Can you work these out from the model? Positions are in its coordinate system, mm. Round coordinates to 2 decimals unless told otherwise and drop trailing zeros.
(1) If I drill on line 1 along Y through (x, z) = (11.6, -881.5) (3 decimals); line 2 along X through (y, z) = (-26.5, -954); line 3 along X through (y, z) = (-21.5, -768), over which ranges is the centre line in solid material (lowest first)?
(2) I want a section at A-A on z = -800. Give the number of separate pieces and of enclosed holes in the cut face, plus the area to 3 significant figures.
(3) Will these pins go through, and if not, where does the flat tip stop? pin 1 Ø0.5 at (x, z) = (13.5, -813) entering from +Y; pin 2 Ø5.5 at (x, y) = (-11.6, -26.625) entering from +Z; pin 3 Ø0.8 at (x, z) = (14, -592) entering from -Y.
from build123d import *

# Parameters (mm, degrees)
SKETCH1_R           = 2.1
SKETCH1_R_2         = 3.4
BOSS_EXTRUDE1_DEPTH = 550


with BuildPart() as part:
    # Sketch1 → Boss-Extrude1 (new body)
    with BuildSketch(Plane(origin=(0, 0, -1000), x_dir=(-1, 0, 0), z_dir=(0, 0, -1))):
        with BuildLine():
            Line((15, -28), (15, -19.3))
            ThreePointArc((15, -19.3), (14.912132034, -19.087867966), (14.7, -19))
            Line((14.7, -19), (13, -19))
            Line((13, -19), (13, -23.25))
            Line((13, -23.25), (9.6642, -23.25))
            Line((9.6642, -23.25), (6, -19.5858))
            Line((6, -19.5858), (6, -15.519615242))
            Line((6, -15.519615242), (5.7, -15))
            Line((5.7, -15), (6, -14.480384758))
            Line((6, -14.480384758), (6, -10.4142))
            Line((6, -10.4142), (9.6642, -6.75))
            Line((9.6642, -6.75), (13, -6.75))
            Line((13, -6.75), (13, -11))
            Line((13, -11), (14.7, -11))
            ThreePointArc((14.7, -11), (14.912132034, -10.912132034), (15, -10.7))
            Line((15, -10.7), (15, 10.7))
            ThreePointArc((15, 10.7), (14.912132034, 10.912132034), (14.7, 11))
            Line((14.7, 11), (13, 11))
            Line((13, 11), (13, 6.75))
            Line((13, 6.75), (9.6642, 6.75))
            Line((9.6642, 6.75), (6, 10.4142))
            Line((6, 10.4142), (6, 14.480384758))
            Line((6, 14.480384758), (5.7, 15))
            Line((5.7, 15), (6, 15.519615242))
            Line((6, 15.519615242), (6, 19.5858))
            Line((6, 19.5858), (9.6642, 23.25))
            Line((9.6642, 23.25), (13, 23.25))
            Line((13, 23.25), (13, 19))
            Line((13, 19), (14.7, 19))
            ThreePointArc((14.7, 19), (14.912132034, 19.087867966), (15, 19.3))
            Line((15, 19.3), (15, 28))
            ThreePointArc((15, 28), (14.414213562, 29.414213562), (13, 30))
            Line((13, 30), (4.3, 30))
            ThreePointArc((4.3, 30), (4.087867966, 29.912132034), (4, 29.7))
            Line((4, 29.7), (4, 28))
            Line((4, 28), (8.25, 28))
            Line((8.25, 28), (8.25, 24.6642))
            Line((8.25, 24.6642), (4.5858, 21))
            Line((4.5858, 21), (0.519615242, 21))
            Line((0.519615242, 21), (0, 20.7))
            Line((0, 20.7), (-0.519615242, 21))
            Line((-0.519615242, 21), (-4.5858, 21))
            Line((-4.5858, 21), (-8.25, 24.6642))
            Line((-8.25, 24.6642), (-8.25, 28))
            Line((-8.25, 28), (-4, 28))
            Line((-4, 28), (-4, 29.7))
            ThreePointArc((-4, 29.7), (-4.087867966, 29.912132034), (-4.3, 30))
            Line((-4.3, 30), (-13, 30))
            ThreePointArc((-13, 30), (-14.414213562, 29.414213562), (-15, 28))
            Line((-15, 28), (-15, 19.3))
            ThreePointArc((-15, 19.3), (-14.912132034, 19.087867966), (-14.7, 19))
            Line((-14.7, 19), (-13, 19))
            Line((-13, 19), (-13, 23.25))
            Line((-13, 23.25), (-9.6642, 23.25))
            Line((-9.6642, 23.25), (-6, 19.5858))
            Line((-6, 19.5858), (-6, 15.519615242))
            Line((-6, 15.519615242), (-5.7, 15))
            Line((-5.7, 15), (-6, 14.480384758))
            Line((-6, 14.480384758), (-6, 10.4142))
            Line((-6, 10.4142), (-9.6642, 6.75))
            Line((-9.6642, 6.75), (-13, 6.75))
            Line((-13, 6.75), (-13, 11))
            Line((-13, 11), (-14.7, 11))
            ThreePointArc((-14.7, 11), (-14.912132034, 10.912132034), (-15, 10.7))
            Line((-15, 10.7), (-15, -10.7))
            ThreePointArc((-15, -10.7), (-14.912132034, -10.912132034), (-14.7, -11))
            Line((-14.7, -11), (-13, -11))
            Line((-13, -11), (-13, -6.75))
            Line((-13, -6.75), (-9.6642, -6.75))
            Line((-9.6642, -6.75), (-6, -10.4142))
            Line((-6, -10.4142), (-6, -14.480384758))
            Line((-6, -14.480384758), (-5.7, -15))
            Line((-5.7, -15), (-6, -15.519615242))
            Line((-6, -15.519615242), (-6, -19.5858))
            Line((-6, -19.5858), (-9.6642, -23.25))
            Line((-9.6642, -23.25), (-13, -23.25))
            Line((-13, -23.25), (-13, -19))
            Line((-13, -19), (-14.7, -19))
            ThreePointArc((-14.7, -19), (-14.912132034, -19.087867966), (-15, -19.3))
            Line((-15, -19.3), (-15, -28))
            ThreePointArc((-15, -28), (-14.414213562, -29.414213562), (-13, -30))
            Line((-13, -30), (-4.3, -30))
            ThreePointArc((-4.3, -30), (-4.087867966, -29.912132034), (-4, -29.7))
            Line((-4, -29.7), (-4, -28))
            Line((-4, -28), (-8.25, -28))
            Line((-8.25, -28), (-8.25, -24.6642))
            Line((-8.25, -24.6642), (-4.5858, -21))
            Line((-4.5858, -21), (-0.519615242, -21))
            Line((-0.519615242, -21), (0, -20.7))
            Line((0, -20.7), (0.519615242, -21))
            Line((0.519615242, -21), (4.5858, -21))
            Line((4.5858, -21), (8.25, -24.6642))
            Line((8.25, -24.6642), (8.25, -28))
            Line((8.25, -28), (4, -28))
            Line((4, -28), (4, -29.7))
            ThreePointArc((4, -29.7), (4.087867966, -29.912132034), (4.3, -30))
            Line((4.3, -30), (13, -30))
            ThreePointArc((13, -30), (14.414213562, -29.414213562), (15, -28))
        make_face()
        with Locations((11.6, 26.625)):
            Circle(SKETCH1_R, mode=Mode.SUBTRACT)
        with Locations((11.6, -26.625)):
            Circle(SKETCH1_R, mode=Mode.SUBTRACT)
        with Locations((0, -15)):
            Circle(SKETCH1_R_2, mode=Mode.SUBTRACT)
        with Locations((0, 15)):
            Circle(SKETCH1_R_2, mode=Mode.SUBTRACT)
        with Locations((-11.6, 26.625)):
            Circle(SKETCH1_R, mode=Mode.SUBTRACT)
        with Locations((-11.6, -26.625)):
            Circle(SKETCH1_R, mode=Mode.SUBTRACT)
        with BuildLine():
            Line((13, 3.75), (13, -3.75))
            ThreePointArc((13, -3.75), (12.707106781, -4.457106781), (12, -4.75))
            Line((12, -4.75), (8.8358, -4.75))
            Line((8.8358, -4.75), (3.476201279, -10.109598721))
            ThreePointArc((3.476201279, -10.109598721), (0, -9), (-3.476201279, -10.109598721))
            Line((-3.476201279, -10.109598721), (-8.8358, -4.75))
            Line((-8.8358, -4.75), (-12, -4.75))
            ThreePointArc((-12, -4.75), (-12.707106781, -4.457106781), (-13, -3.75))
            Line((-13, -3.75), (-13, 3.75))
            ThreePointArc((-13, 3.75), (-12.707106781, 4.457106781), (-12, 4.75))
            Line((-12, 4.75), (-8.8358, 4.75))
            Line((-8.8358, 4.75), (-3.476201279, 10.109598721))
            ThreePointArc((-3.476201279, 10.109598721), (0, 9), (3.476201279, 10.109598721))
            Line((3.476201279, 10.109598721), (8.8358, 4.75))
            Line((8.8358, 4.75), (12, 4.75))
            ThreePointArc((12, 4.75), (12.707106781, 4.457106781), (13, 3.75))
        make_face(mode=Mode.SUBTRACT)
    extrude(amount=-BOSS_EXTRUDE1_DEPTH)


solid = part.part
Filled sheet:
1. line 1: y = -30 to -28.725, -24.525 to -23.25, -6.75 to -4.75, 4.75 to 6.75, 23.25 to 24.525, 28.725 to 30
1. line 2: x = -15 to -13.7, -9.5 to -8.25, 8.25 to 9.5, 13.7 to 15
1. line 3: x = -15 to -13, -7.91 to -5.09, 5.09 to 7.91, 13 to 15
2. separate pieces: 1
2. enclosed holes: 7
2. area: 591 mm2
3. pin 1: stops at y = 29.98
3. pin 2: stops at z = -450
3. pin 3: stops at y = -29.91
